from build123d import *

# Parameters (mm, degrees)
EXTRUDE_1_DEPTH     = 20
SKETCH_4_W          = 20
SKETCH_4_H          = 16.999999963
CUT_EXTRUDE_1_DEPTH = 47.935226042
SKETCH_6_W          = 30.048551437
SKETCH_6_H          = 22.650000031
EXTRUDE_1_2_DEPTH   = 2
SKETCH_7_R          = 2.5
CUT_EXTRUDE_2_DEPTH = 53.675836409


with BuildPart() as part:
    # Эскиз1 → Extrude 1 (new body)
    with BuildSketch(Plane.XY):
        Polygon((0, 30), (0, 0), (-28.048551439, 0), (-28.048551439, -2), (2, -2), (2, 30), align=None)
    extrude(amount=EXTRUDE_1_DEPTH)

    # Эскиз4 → Вырез-Вытянуть1 (cut, through all)
    with BuildSketch(Plane(origin=(2, 0, 0), x_dir=(0, 0, -1), z_dir=(1, 0, 0))):
        with Locations((-10, 21.500000019)):
            Rectangle(SKETCH_4_W, SKETCH_4_H)
    extrude(amount=-CUT_EXTRUDE_1_DEPTH, mode=Mode.SUBTRACT)

    # Эскиз6 → Extrude 1 2 (add)
    with BuildSketch(Plane(origin=(0, 0, 0), x_dir=(1, 0, 0), z_dir=(0, 1, 0))):
        Polygon((-28.048551439, 0), (1.999999998, 0), (2.000000002, 22.349999969), (-28.048551439, 22.349999969), align=None)
        with Locations((-13.024275721, -31.325000016)):
            Rectangle(SKETCH_6_W, SKETCH_6_H)
    extrude(amount=-EXTRUDE_1_2_DEPTH)

    # Эскиз7 → Вырез-Вытянуть2 (cut, through all)
    with BuildSketch(Plane(origin=(0, 0, 0), x_dir=(1, 0, 0), z_dir=(0, 1, 0))):
        with Locations(Location((-12.999999999, 6.09999997, 0), (0, 0, 270))):
            Circle(SKETCH_7_R)
        with Locations(Location((-13.000000001, -26.40000003, 0), (0, 0, 270))):
            Circle(SKETCH_7_R)
    extrude(amount=-CUT_EXTRUDE_2_DEPTH, mode=Mode.SUBTRACT)


solid = part.part
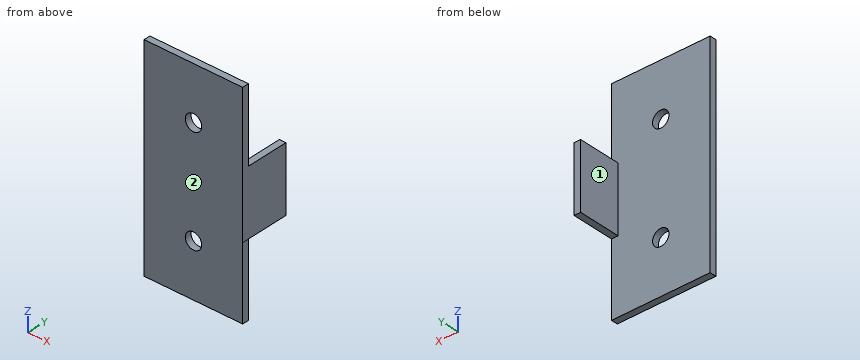
For this review, take the finished solid that the model builds, in its own axes (mm). Face numbers are marked on the shaded views. A direction names the side the tool comes from. Round coordinates to 2 decimals unless told otherwise and drop trailing zeros. Order: outer loops, then holes, each group sorted by start corner. A loop starts at its lowest first (then second) coordinate and runs counter-clockwise, first axis right, second up. Notation, with made-up numbers: (32, 87.25) -> (79, 87.25) arc R26 cw to (79, 118.25) -> close; hole circle Ø6 at (41, 54.5). An arc over 180 degrees is marked (long way). Write item = value, one per line. Start each with the question number.
1) Take a section at B-B on z = -6.1. State the section outline as (x, y) points.
2) Take a section at D-D on y = 3.5. State the section outline as (x, z) points.
3) Take a section at C-C on z = 18.5. State the section outline as (x, y) points.
4) To check wall thickness, follow line 1 (X direction, y = -1, z = -6.1); line 2 (X direction, y = 6.5, z = 8); line 3 (Y direction, x = -27, z = 5). State the ranges of each line that lie inside material, in increasing order. Write a range as from..to.
5) Take a section at A-A on x = -11.5. State the section outline as (y, z) points.
6) Insertion check: pin 1 (5 mm diameter, centred on x = -10, z = 20.5, fed in from +Y); pin 2 (1.6 mm diameter, centred on x = 1, y = 5, fed in from -Z); pin 3 (4 mm diameter, centred on y = 4, z = 5, fed in from -X). Each pin has a flat end and moves straight along its axis. Give the tip position at first contact, or say it passes through.
7) Tool access review of the marked faces 1 and 2: name each direction out of +Z, -Z, +X, -X, +Y, -Y from which nothing blocks a thin tool from reaching the whole face with its end or side.
Verdict:
q1.outline = (-28.05, -2) -> (-15.5, -2) -> (-15.5, 0) -> (-28.05, 0) -> close; (-10.5, -2) -> (2, -2) -> (2, 0) -> (-10.5, 0) -> close
q2.outline = (0, 0) -> (2, 0) -> (2, 20) -> (0, 20) -> close
q3.outline = (-28.05, -2) -> (2, -2) -> (2, 13) -> (0, 13) -> (0, 0) -> (-28.05, 0) -> close
q4.line_1 = -28.05..-15.5, -10.5..2
q4.line_2 = 0..2
q4.line_3 = -2..0
q5.outline = (-2, -22.35) -> (0, -22.35) -> (0, -8.1) -> (-2, -8.1) -> close; (-2, -4.1) -> (0, -4.1) -> (0, 24.4) -> (-2, 24.4) -> close; (-2, 28.4) -> (0, 28.4) -> (0, 42.65) -> (-2, 42.65) -> close
q6.pin_1 = 0
q6.pin_2 = 0
q6.pin_3 = 0
q7.face_1 = +Z, -Z, -X, +Y
q7.face_2 = +Z, -Z, +X, -X, -Y
